from build123d import *

# Parameters (mm, degrees)
SKETCH1_R           = 2.5
BOSS_EXTRUDE2_DEPTH = 4
FILLET1_R           = 5
FILLET2_R           = 3
FILLET3_R           = 3
BOSS_EXTRUDE3_START = -47
SKETCH2_R           = 2.5
BOSS_EXTRUDE3_DEPTH = 47
FILLET4_R           = 20
CUT_EXTRUDE1_REACH  = 115.914
SKETCH3_W           = 6
SKETCH3_H           = 11
SKETCH4_W           = 4
SKETCH4_H           = 23
BOSS_EXTRUDE4_DEPTH = 3
FILLET5_START       = -50
FILLET5_DEPTH       = 4
FILLET5_START_2     = 46
FILLET5_2_DEPTH     = 4
SKETCH5_W           = 23
SKETCH5_H           = 4
BOSS_EXTRUDE5_DEPTH = 3
FILLET6_START       = -25
FILLET6_DEPTH       = 4
SKETCH6_W           = 23
SKETCH6_H           = 4
BOSS_EXTRUDE6_DEPTH = 3
FILLET7_START       = -25
FILLET7_DEPTH       = 4


with BuildPart() as part:
    # Sketch1 → Boss-Extrude2 (new body)
    with BuildSketch(Plane.XY):
        Polygon((-50, -25), (-41.75, -25), (41.75, -25), (50, -25), (50, -16.75), (50, 16.75), (50, 25), (41.75, 25), (-50, 25), (-50, -16.75), align=None)
        with Locations((-45, -20)):
            Circle(SKETCH1_R, mode=Mode.SUBTRACT)
        with Locations((45, -20)):
            Circle(SKETCH1_R, mode=Mode.SUBTRACT)
        with BuildLine():
            Line((-45, -16.75), (-46, -16.75))
            Line((-46, -16.75), (-46, 21))
            Line((-46, 21), (41.75, 21))
            Line((41.75, 21), (41.75, 20))
            ThreePointArc((41.75, 20), (42.701902961, 17.701902961), (45, 16.75))
            Line((45, 16.75), (46, 16.75))
            Line((46, 16.75), (46, -16.75))
            Line((46, -16.75), (45, -16.75))
            ThreePointArc((45, -16.75), (42.701902961, -17.701902961), (41.75, -20))
            Line((41.75, -20), (41.75, -21))
            Line((41.75, -21), (-41.75, -21))
            Line((-41.75, -21), (-41.75, -20))
            ThreePointArc((-41.75, -20), (-42.701902961, -17.701902961), (-45, -16.75))
        make_face(mode=Mode.SUBTRACT)
        with Locations((45, 20)):
            Circle(SKETCH1_R, mode=Mode.SUBTRACT)
    extrude(amount=BOSS_EXTRUDE2_DEPTH)

    # Fillet1
    fillet1_edges = [part.edges().sort_by_distance(p)[0] for p in [
        (50, 25, 2),
        (50, -25, 2),
        (-50, -25, 2),
    ]]
    fillet(fillet1_edges, radius=FILLET1_R)

    # Fillet2
    fillet2_edges = [part.edges().sort_by_distance(p)[0] for p in [
        (41.75, 21, 2),
        (46, 16.75, 2),
        (46, -16.75, 2),
        (41.75, -21, 2),
        (-41.75, -21, 2),
        (-46, -16.75, 2),
    ]]
    fillet(fillet2_edges, radius=FILLET2_R)

    # Fillet3
    fillet3_edges = [part.edges().sort_by_distance(p)[0] for p in [
        (-46, 21, 2),
        (-50, 25, 2),
    ]]
    fillet(fillet3_edges, radius=FILLET3_R)

    # Sketch2 → Boss-Extrude3 (add)
    # profile 1 of 2: a face of its own
    with BuildSketch(Plane.XY.offset(4).offset(BOSS_EXTRUDE3_START)):
        with BuildLine():
            Line((-46, -14.078640359), (-50, -14.078640359))
            Line((-50, -14.078640359), (-50, -16.75))
            Line((-50, -16.75), (-50, -20))
            ThreePointArc((-50, -20), (-48.535533906, -23.535533906), (-45, -25))
            Line((-45, -25), (-41.75, -25))
            Line((-41.75, -25), (-39.078640359, -25))
            Line((-39.078640359, -25), (-39.078640359, -21))
            ThreePointArc((-39.078640359, -21), (-40.827925927, -20.437211521), (-41.920892987, -18.96))
            ThreePointArc((-41.920892987, -18.96), (-42.701902961, -17.701902961), (-43.96, -16.920892987))
            ThreePointArc((-43.96, -16.920892987), (-45.437211521, -15.827925927), (-46, -14.078640359))
        make_face()
        with Locations((-45, -20)):
            Circle(SKETCH2_R, mode=Mode.SUBTRACT)
    # profile 2 of 2: a face of its own
    with BuildSketch(Plane.XY.offset(4).offset(BOSS_EXTRUDE3_START)):
        with BuildLine():
            Line((39.078640359, -21), (39.078640359, -25))
            Line((39.078640359, -25), (45, -25))
            ThreePointArc((45, -25), (48.535533906, -23.535533906), (50, -20))
            Line((50, -20), (50, -14.078640359))
            Line((50, -14.078640359), (46, -14.078640359))
            ThreePointArc((46, -14.078640359), (45.437211521, -15.827925927), (43.96, -16.920892987))
            ThreePointArc((43.96, -16.920892987), (42.701902961, -17.701902961), (41.920892987, -18.96))
            ThreePointArc((41.920892987, -18.96), (40.827925927, -20.437211521), (39.078640359, -21))
        make_face()
        with Locations((45, -20)):
            Circle(SKETCH2_R, mode=Mode.SUBTRACT)
    extrude(amount=BOSS_EXTRUDE3_DEPTH)

    # Fillet4
    # the kernel refuses this fillet: 20 mm, written as the material it adds along each edge
    with BuildSketch(Plane(origin=(-50, -14.078640359, 0), x_dir=(0, 1, 0), z_dir=(1, 0, 0)), Plane(origin=(39.078640359, -25, 0), x_dir=(-1, 0, 0), z_dir=(0, 1, 0))) as fillet4_piece_1:
        with BuildLine():
            CenterArc((FILLET4_R, -FILLET4_R), FILLET4_R, 90, 90)
            Line((0, -FILLET4_R), (0, 0))
            Line((0, 0), (FILLET4_R, 0))
        make_face()
    extrude(amount=4)
    with BuildSketch(Plane(origin=(-39.078640359, -21, 0), x_dir=(0, 0, -1), z_dir=(0, -1, 0)), Plane(origin=(46, -14.078640359, 0), x_dir=(0, 0, -1), z_dir=(1, 0, 0))) as fillet4_piece_2:
        with BuildLine():
            CenterArc((FILLET4_R, FILLET4_R), FILLET4_R, 180, 90)
            Line((0, FILLET4_R), (0, 0))
            Line((0, 0), (FILLET4_R, 0))
        make_face()
    extrude(amount=4)

    # Sketch3 → Cut-Extrude1 (cut, up to next)
    with BuildSketch(Plane(origin=(-36.035533906, -36.035533906, 0), x_dir=(0, 0, -1), z_dir=(0.707106781186548, 0.7071067811865471, 0)), mode=Mode.PRIVATE) as cut_extrude1_sk1:
        with Locations((4, 17.67766953)):
            Rectangle(SKETCH3_W, SKETCH3_H)
    cut_extrude1_tool1 = extrude(cut_extrude1_sk1.sketch, amount=CUT_EXTRUDE1_REACH, mode=Mode.PRIVATE) & part.part
    # Sketch3 → Cut-Extrude1 (cut, up to next)
    with BuildSketch(Plane(origin=(-36.035533906, -36.035533906, 0), x_dir=(0, 0, -1), z_dir=(0.707106781186548, 0.7071067811865471, 0)), mode=Mode.PRIVATE) as cut_extrude1_sk2:
        with Locations((36, 17.67766953)):
            Rectangle(SKETCH3_W, SKETCH3_H)
    cut_extrude1_tool2 = extrude(cut_extrude1_sk2.sketch, amount=CUT_EXTRUDE1_REACH, mode=Mode.PRIVATE) & part.part
    cut_extrude1_1 = cut_extrude1_tool1.solids().sort_by_distance((-48.535534, -23.535534, -4))[0]
    add(cut_extrude1_1, mode=Mode.SUBTRACT)
    cut_extrude1_2 = cut_extrude1_tool2.solids().sort_by_distance((-48.535534, -23.535534, -36))[0]
    add(cut_extrude1_2, mode=Mode.SUBTRACT)
    cut_extrude1 = cut_extrude1_1 + cut_extrude1_2  # Cut-Extrude1 as one shape, for the pattern or mirror that repeats it

    # Mirror1: Cut-Extrude1 across plane
    add(cut_extrude1.mirror(Plane(origin=(0, 0, 0), x_dir=(0, 0, 1), z_dir=(1, 0, 0))), mode=Mode.SUBTRACT)

    # Sketch4 → Boss-Extrude4 (add)
    with BuildSketch(Plane(origin=(0, -14.078640359, 0), x_dir=(1, 0, 0), z_dir=(0, 1, 0))):
        with Locations((-48, 31.5)):
            Rectangle(SKETCH4_W, SKETCH4_H)
        with Locations((48, 31.5)):
            Rectangle(SKETCH4_W, SKETCH4_H)
    extrude(amount=BOSS_EXTRUDE4_DEPTH)

    # Fillet5: read off the stored shape, not the designer's step
    # Fillet5 outline → Fillet5 (add)
    with BuildSketch(Plane.YZ.offset(FILLET5_START)):
        with BuildLine():
            ThreePointArc((-11.078640359, -20), (-10.703206123, -10.372818577), (-4.549228594, -2.959847946))
            ThreePointArc((-4.549228594, -2.959847946), (-11.534466961, -10.238129398), (-14.078640359, -20))
            Line((-14.078640359, -20), (-11.078640359, -20))
        make_face()
    extrude(amount=FILLET5_DEPTH)

    # Fillet5 2 outline → Fillet5 2 (add)
    with BuildSketch(Plane.YZ.offset(FILLET5_START_2)):
        with BuildLine():
            ThreePointArc((-11.078640359, -20), (-10.703206123, -10.372818577), (-4.549228594, -2.959847946))
            ThreePointArc((-4.549228594, -2.959847946), (-11.534466961, -10.238129398), (-14.078640359, -20))
            Line((-14.078640359, -20), (-11.078640359, -20))
        make_face()
    extrude(amount=FILLET5_2_DEPTH)

    # Sketch5 → Boss-Extrude5 (add)
    with BuildSketch(Plane(origin=(-39.078640359, 0, 0), x_dir=(0, 0, -1), z_dir=(1, 0, 0))):
        with Locations((31.5, -23)):
            Rectangle(SKETCH5_W, SKETCH5_H)
    extrude(amount=BOSS_EXTRUDE5_DEPTH)

    # Fillet6: read off the stored shape, not the designer's step
    # Fillet6 outline → Fillet6 (add)
    with BuildSketch(Plane(origin=(0, 0, 0), x_dir=(1, 0, 0), z_dir=(0, 1, 0)).offset(FILLET6_START)):
        with BuildLine():
            ThreePointArc((-39.078640359, 20), (-36.534466961, 10.238129398), (-29.549228594, 2.959847946))
            ThreePointArc((-29.549228594, 2.959847946), (-35.703206123, 10.372818577), (-36.078640359, 20))
            Line((-36.078640359, 20), (-39.078640359, 20))
        make_face()
    extrude(amount=FILLET6_DEPTH)

    # Sketch6 → Boss-Extrude6 (add)
    with BuildSketch(Plane.ZY.offset(-39.078640359)):
        with Locations((-31.5, -23)):
            Rectangle(SKETCH6_W, SKETCH6_H)
    extrude(amount=BOSS_EXTRUDE6_DEPTH)

    # Fillet7: read off the stored shape, not the designer's step
    # Fillet7 outline → Fillet7 (add)
    with BuildSketch(Plane(origin=(0, 0, 0), x_dir=(1, 0, 0), z_dir=(0, 1, 0)).offset(FILLET7_START)):
        with BuildLine():
            ThreePointArc((36.078640359, 20), (35.703206123, 10.372818577), (29.549228594, 2.959847946))
            ThreePointArc((29.549228594, 2.959847946), (36.534466961, 10.238129398), (39.078640359, 20))
            Line((39.078640359, 20), (36.078640359, 20))
        make_face()
    extrude(amount=FILLET7_DEPTH)


solid = part.part
Work out the finished part from the listing and answer in its coordinate system (mm). A direction names the side the tool comes from. Give positions to 0.01 mm unless a question says otherwise; leave off trailing zeros. Write each loop counter-clockwise with the first axis right and the second up, starting at its lowest first coordinate (ties: lowest second). Pieces come first, ordered by that corner, then holes. Notation, with made-up numbers: M -1,-0.5 L 51,-0.5 A13 cw 51,11.5 Z; hole C 6,-33.75 d6. An arc over 180 degrees is marked long. Answer as CSV lines item,"result".
Q1. A tool of negligible diameter and unlimited length cuts with its end or side. For faces 5 (the cylindrical face through (42.717, -17.687, 1.465)), 6 (the flat face through (40.67, -23.45, -35.96)), 7 (the cylindrical face through (-40.81, -20.45, -41.03)), 8 (the flat face through (-47, -22, -33)), 9 (the flat face through (-48.03, -15.25, -3.96)), from which of +Z, -Z, +X, -X, +Y, -Y can it reach the whole face along a straight path? Write none if from no direction.
A:
face 5,"+Z, -Z"
face 6,"+X, +Y"
face 7,"+Z, -Z, +Y"
face 8,"none"
face 9,"-Y"
Q2. A cutting plane is placed at C-C on z = -12. Write down the section's boundary in (x, y), plus the area to 3 significant figures.
A:
outline,"M -50,-20 A5 ccw -45,-25 L -36.22,-25 L -36.22,-21 L -39.08,-21 A3 cw -41.92,-18.96 A3.25 ccw -43.96,-16.92 A3 cw -46,-14.08 L -46,-11.22 L -50,-11.22 Z; M 36.22,-25 L 45,-25 A5 ccw 50,-20 L 50,-11.22 L 46,-11.22 L 46,-14.08 A3 cw 43.96,-16.92 A3.25 ccw 41.92,-18.96 A3 cw 39.08,-21 L 36.22,-21 Z; hole C -45,-20 d5; hole C 45,-20 d5"
area,"175 mm²"
Q3. The mould has two halves that part along Z. Classify faces 1 (the cylindrical face through (49, 23, 2)), 2 (the flat face through (0, 22, 0)), 3 (the flat face through (0, -22, 4)), 4 (the flat face through (-47, -22, -1)): +Z half, -Z half, draft (parallel to the pull), parting line (faces both ways), or undercut.
A:
face 1,"draft"
face 2,"-Z half"
face 3,"+Z half"
face 4,"undercut"
Q4. Find the intervals of material crossed by probe 1 along Y at (x, z) = (45, 2); probe 2 along X at (y, z) = (-20, -22.5); probe 3 along Y at (x, z) = (45, -27), in increasing order. Write a range as [from, to].
A:
probe 1,"y = [-25, -22.5], [-17.5, -16.31], [16.31, 17.5], [22.5, 25]"
probe 2,"x = [-50, -47.5], [-42.5, -41.31], [41.31, 42.5], [47.5, 50]"
probe 3,"y = [-25, -22.5], [-17.5, -16.31]"
Q5. A cutting plane is placed at D-D on x = -33. Write down the section's boundary in (y, z).
A:
outline,"M -25,-5.88 L -21,-5.88 L -21,4 L -25,4 Z; M 21,0 L 25,0 L 25,4 L 21,4 Z"
Q6. A cutting plane is placed at B-B on x = -3. Write down the section's boundary in (y, z).
A:
outline,"M -25,0 L -21,0 L -21,4 L -25,4 Z; M 21,0 L 25,0 L 25,4 L 21,4 Z"
Q7. A cutting plane is placed at A-A on z = -25.5. Write down the section's boundary in (x, y).
A:
outline,"M -50,-20 A5 ccw -45,-25 L -36.08,-25 L -36.08,-21 L -39.08,-21 A3 cw -41.92,-18.96 A3.25 ccw -43.96,-16.92 A3 cw -46,-14.08 L -46,-11.08 L -50,-11.08 Z; M 36.08,-25 L 45,-25 A5 ccw 50,-20 L 50,-11.08 L 46,-11.08 L 46,-14.08 A3 cw 43.96,-16.92 A3.25 ccw 41.92,-18.96 A3 cw 39.08,-21 L 36.08,-21 Z; hole C -45,-20 d5; hole C 45,-20 d5"
Q8. Given P1, Ø2, axis at x = -1, y = -24, coming from the -Z side; P2, Ø6, axis at x = -45, y = -20, coming from the +Z side; P3, Ø3, axis at x = 49, z = -32, coming from the +Y side; P4, Ø4.5, axis at y = -23, z = -32, coming from the -X side, each flat-ended and moving along its own axis, determine where each tip first touches the part or whether it passes through.
A:
P1,"stops at z = 0"
P2,"stops at z = 4"
P3,"stops at y = -11.08"
P4,"stops at x = -49.94"
